Part model, mm, in its own coordinate system. A direction names the side the tool comes from. Give positions to 0.01 mm unless a question says otherwise; leave off trailing zeros. Order: outer loops, then holes, each group sorted by start corner. A loop starts at its lowest first (then second) coordinate and runs counter-clockwise, first axis right, second up. Notation, with made-up numbers: (0, 54) - (35, 54) arc R23 ccw to (35, 78) - close; hole circle Ø4 at (-15, 13.25). An arc over 180 degrees is marked (long way). One line per item, written item: value.
```python
from build123d import *

# Parameters (mm, degrees)
SKETCH1_R           = 11.1125
BOSS_EXTRUDE1_DEPTH = 19.05
SKETCH2_R           = 14.2875
BOSS_EXTRUDE2_DEPTH = 12.7
CUT_EXTRUDE1_START  = -8.89
SKETCH3_R           = 14.2875
CUT_EXTRUDE1_DEPTH  = 8.89
CHAMFER1_SIZE       = 1.27
CUT_EXTRUDE2_REACH  = 39.634
SKETCH4_R           = 1


with BuildPart() as part:
    # Sketch1 → Boss-Extrude1 (new body)
    with BuildSketch(Plane.XY):
        with Locations(Location((0, 0, 0), (0, 0, 180))):
            Circle(SKETCH1_R)
    extrude(amount=BOSS_EXTRUDE1_DEPTH)

    # Sketch2 → Boss-Extrude2 (add)
    with BuildSketch(Plane.XY.offset(19.05)):
        Circle(SKETCH2_R)
    extrude(amount=BOSS_EXTRUDE2_DEPTH)

    # Sketch3 → Cut-Extrude1 (cut)
    with BuildSketch(Plane.XY.offset(31.75).offset(CUT_EXTRUDE1_START)):
        Circle(SKETCH3_R)
        Polygon((12.831609733, 0), (6.415804866, 11.1125), (-6.415804866, 11.1125), (-12.831609733, 0), (-6.415804866, -11.1125), (6.415804866, -11.1125), align=None, mode=Mode.SUBTRACT)
    extrude(amount=CUT_EXTRUDE1_DEPTH, mode=Mode.SUBTRACT)

    # Chamfer1
    chamfer1_edges = [part.edges().sort_by_distance(p)[0] for p in [
        (-14.2875, 0, 22.86),
    ]]
    chamfer(chamfer1_edges, length=CHAMFER1_SIZE)

    # Cut-Loft1: read off the stored shape, not the designer's step
    # Cut-Loft1: loft between two sections, ruled curve by curve
    cut_loft1_from = [
        Edge.make_bspline([(2.35183174, 9.256296648, 0), (-16.160761555, 13.959960127, 0), (-20.864425035, -4.552633168, 0), (-2.35183174, -9.256296648, 0), (16.160761555, -13.959960127, 0), (20.864425035, 4.552633168, 0), (2.35183174, 9.256296648, 0)], [0, 0, 0, 0, 0.5, 0.5, 0.5, 1, 1, 1, 1], 3, [1, 0.333333333, 0.333333333, 1, 0.333333333, 0.333333333, 1]),
    ]
    cut_loft1_to = [
        Edge.make_bspline([(2.644109425, 4.759906548, 22.86), (-6.875703672, 10.048125398, 22.86), (-12.163922522, 0.528312301, 22.86), (-2.644109425, -4.759906548, 22.86), (6.875703672, -10.048125398, 22.86), (12.163922522, -0.528312301, 22.86), (2.644109425, 4.759906548, 22.86)], [0, 0, 0, 0, 0.5, 0.5, 0.5, 1, 1, 1, 1], 3, [1, 0.333333333, 0.333333333, 1, 0.333333333, 0.333333333, 1]),
    ]
    cut_loft1 = Solid(Shell([*[Face.make_surface_from_curves(cut_loft1_from[k], cut_loft1_to[k]) for k in range(1)], Face(Wire(cut_loft1_from)), Face(Wire(cut_loft1_to))]))
    add(cut_loft1, mode=Mode.SUBTRACT)

    # Sketch4 → Cut-Extrude2 (cut, up to next)
    with BuildSketch(Plane.XY.offset(31.75), mode=Mode.PRIVATE) as cut_extrude2_sk1:
        with Locations((0, 4.445)):
            Circle(SKETCH4_R)
    cut_extrude2_tool1 = extrude(cut_extrude2_sk1.sketch, amount=-CUT_EXTRUDE2_REACH, mode=Mode.PRIVATE) & part.part
    # Sketch4 → Cut-Extrude2 (cut, up to next)
    with BuildSketch(Plane.XY.offset(31.75), mode=Mode.PRIVATE) as cut_extrude2_sk2:
        with Locations((3.84948292, -2.2225)):
            Circle(SKETCH4_R)
    cut_extrude2_tool2 = extrude(cut_extrude2_sk2.sketch, amount=-CUT_EXTRUDE2_REACH, mode=Mode.PRIVATE) & part.part
    # Sketch4 → Cut-Extrude2 (cut, up to next)
    with BuildSketch(Plane.XY.offset(31.75), mode=Mode.PRIVATE) as cut_extrude2_sk3:
        with Locations((-3.84948292, -2.2225)):
            Circle(SKETCH4_R)
    cut_extrude2_tool3 = extrude(cut_extrude2_sk3.sketch, amount=-CUT_EXTRUDE2_REACH, mode=Mode.PRIVATE) & part.part
    add(cut_extrude2_tool1.solids().sort_by_distance((0, 4.445, 31.75))[0], mode=Mode.SUBTRACT)
    add(cut_extrude2_tool2.solids().sort_by_distance((3.849483, -2.2225, 31.75))[0], mode=Mode.SUBTRACT)
    add(cut_extrude2_tool3.solids().sort_by_distance((-3.849483, -2.2225, 31.75))[0], mode=Mode.SUBTRACT)


solid = part.part
```
1) Drill centre lines: line 1 along Y through (x, z) = (0, 29.75) (1 decimal); line 2 along X through (y, z) = (-2, 25); line 3 along Y through (x, z) = (-2.5, 8.5). Where is each one in solid material? Low to high. Write a range as from..to.
Outcome:
line 1: y = -11.1..3.4, 5.4..11.1
line 2: x = -11.68..-4.82, -2.87..2.87, 4.82..11.68
line 3: y = -10.83..-7.57, 7.57..10.83
2) Pin check, flat tips, straight feed: pin 1 (2 mm diameter, centred on x = -7.5, z = 12, fed in from -Y); pin 2 (3 mm diameter, centred on x = -1.5, z = 27.5, fed in from -Y); pin 3 (10 mm diameter, centred on x = 2.5, z = 27.5, fed in from -Y); pin 4 (1.6 mm diameter, centred on x = -3.85, y = -2.22, fed in from +Z). Stop position of each tip, or through.
Outcome:
pin 1: stops at y = -9.01
pin 2: stops at y = -11.11
pin 3: stops at y = -13.21
pin 4: passes through
3) Which spindle directions (+Z, -Z, +X, -X, +Y, -Y) get a long thin tool onto all of the face, cutting with end or side? Do faces 4 (the flat face through (0, 11.112, 27)), 5 (the flat face through (-9.67, -5.48, 27.24)), 6 (the flat face through (10, -6, 22.86)), 7 (the flat face through (9.67, 5.48, 27.24)), 8 (the flat face through (-9, -7, 19.05)). Say none if no direction does.
Outcome:
face 4: +Z, +X, -X, +Y
face 5: +Z, -X, -Y
face 6: +Z
face 7: +Z, +X, +Y
face 8: -Z
4) Cut at A-A, the plane z = 24.5. Give the cut face in (x, y) (1 decimal), then the cut area to 3 significant figures.
Outcome:
outline: (-12.8, 0) - (-6.4, -11.1) - (6.4, -11.1) - (12.8, 0) - (6.4, 11.1) - (-6.4, 11.1) - close; hole circle Ø2 at (-3.8, -2.2); hole circle Ø2 at (0, 4.4); hole circle Ø2 at (3.8, -2.2)
area: 418 mm^2
5) Mould opens along Y. For faces 1 (the flat face through (-9.6, 5.6, 27.2)), 2 (the flat face through (0, 0, 22.86)), 3 (the flat face through (9.6, -5.6, 27.2)) say: released by +Y, released by -Y, zero draft, split by the parting line, or undercut.
Outcome:
face 1: released by +Y
face 2: undercut
face 3: released by -Y
